```python
from build123d import *

# Parameters (mm, degrees)
F0_R     = 1.5875
F1_DEPTH = 1.778
F3_DEPTH = 9.525


with BuildPart() as f1:
    # F0 (on Top) → F1 (new body)
    with BuildSketch(Plane.XY):
        with BuildLine():
            Line((0, 53.34), (0, 0))
            Line((0, 0), (66.04, 0))
            Line((66.04, 0), (66.04, 2.54))
            Line((66.04, 2.54), (66.04, 6.0325))
            ThreePointArc((66.04, 6.0325), (64.4525, 7.62), (66.04, 9.2075))
            ThreePointArc((66.04, 9.2075), (67.1625320151, 8.7425320151), (67.6275, 7.62))
            Line((67.6275, 7.62), (68.58, 7.62))
            Line((68.58, 7.62), (68.58, 37.846))
            Line((68.58, 37.846), (66.04, 40.386))
            Line((66.04, 40.386), (66.04, 51.816))
            Line((66.04, 51.816), (64.516, 53.34))
            Line((64.516, 53.34), (0, 53.34))
        make_face()
        with Locations((13.97, 2.54)):
            Circle(F0_R, mode=Mode.SUBTRACT)
        with BuildLine():
            ThreePointArc((13.6525, 50.8), (15.24, 52.3875), (16.8275, 50.8))
            ThreePointArc((16.8275, 50.8), (15.24, 49.2125), (13.6525, 50.8))
        make_face(mode=Mode.SUBTRACT)
        with BuildLine():
            ThreePointArc((67.6275, 34.1701958202), (67.1625320151, 33.0476638051), (66.04, 32.5826958202))
            ThreePointArc((66.04, 32.5826958202), (64.9174679849, 35.2927278354), (67.6275, 34.1701958202))
        make_face(mode=Mode.SUBTRACT)
        with BuildLine():
            Line((66.04, 6.0325), (66.04, 2.54))
            Line((66.04, 2.54), (68.58, 5.08))
            Line((68.58, 5.08), (68.58, 7.62))
            Line((68.58, 7.62), (67.6275, 7.62))
            ThreePointArc((67.6275, 7.62), (67.1625320151, 6.4974679849), (66.04, 6.0325))
        make_face()
    extrude(amount=F1_DEPTH)

    # F2 (on face) → F3 (join)
    with BuildSketch(Plane.XY.offset(1.778)):
        Polygon((0, 32.385), (9.525, 32.385), (9.525, 45.085), (-6.35, 45.085), (-6.35, 32.385), align=None)
        Polygon((0, 3.175), (11.43, 3.175), (11.43, 12.065), (-1.905, 12.065), (-1.905, 3.175), align=None)
    extrude(amount=F3_DEPTH)


solid = f1.part
```
Geometry: final body of the model. Coordinates: model frame, mm. A direction names the side the tool comes from. Round coordinates to 2 decimals unless told otherwise and drop trailing zeros. Order: outer loops, then holes, each group sorted by start corner. A loop starts at its lowest first (then second) coordinate and runs counter-clockwise, first axis right, second up. Notation, with made-up numbers: (52, 31) - (62, 31) arc R7 cw to (62, 35) - close; hole circle Ø8 at (58.25, 46). An arc over 180 degrees is marked (long way). Write item = value, one per line. Start each with the question number.
Q1. Pull-direction query (Y, two-part tool) for faces 5 (the flat face through (1, 32.385, 6)), 6 (the flat face through (1, 39, 11.303)), 7 (the flat face through (5, 12.065, 6)), 8 (the flat face through (67.328, 39.098, 0.877)); classes: +Y half, -Y half, draft (parallel to the pull), parting line (faces both ways), or undercut.
Q2. Cut plane D-D on z = 1. Return the cut outline in (x, y) (1 decimal).
Q3. Ray query, line 1 (X direction, y = 50.8, z = 1.45); line 2 (Y direction, x = 13.97, z = 0.9); line 3 (X direction, y = 10, z = 4) (3 decimals). Return the intervals inside material, ascending. Write a range as from..to.
Q4. Access query for faces 1 (the flat face through (9.525, 39, 6)), 2 (the flat face through (5, 3.175, 6)), 3 (the flat face through (-3, 39, 1.778)), 4 (the flat face through (66.04, 1, 1)). Directions: +Z, -Z, +X, -X, +Y, -Y. A direction counts if a zero-diameter tool reaches every point of the face in a straight line with its end or side. Return the directions, or none.
Q5. Pin query (flat end, axial travel): pin 1 (2 mm diameter, centred on y = 47, z = 0.5, fed in from +X); pin 2 (0.9 mm diameter, centred on y = 24, z = 1, fed in from -X); pin 3 (3 mm diameter, centred on x = -3, y = 35.5, fed in from -Z). Return the tip coordinate at first contact, or that it passes through.
Q6. Cut plane B-B on z = 4.5. Return the cut outline in (x, y) (3 decimals), and give its area (3 significant figures).
Q7. Cut plane C-C on y = 43. Return the cut outline in (x, z) (3 decimals), and give its area (3 significant figures).
Q8. Cut plane A-A on y = 50.8. Return the cut outline in (x, z).
Outcome:
q1.face_5 = undercut
q1.face_6 = draft
q1.face_7 = undercut
q1.face_8 = +Y half
q2.outline = (0, 0) - (66, 0) - (66, 2.5) - (68.6, 5.1) - (68.6, 37.8) - (66, 40.4) - (66, 51.8) - (64.5, 53.3) - (0, 53.3) - close; hole circle Ø3.2 at (14, 2.5); hole circle Ø3.2 at (15.2, 50.8); hole circle Ø3.2 at (66, 7.6); hole circle Ø3.2 at (66, 34.2)
q3.line_1 = 0..13.65, 16.83..66.04
q3.line_2 = 0..0.95, 4.13..49.85, 51.75..53.34
q3.line_3 = -1.905..11.43
q4.face_1 = +Z, +X, +Y
q4.face_2 = +Z, +X, -X, -Y
q4.face_3 = -Z, -X, +Y, -Y
q4.face_4 = +Z, -Z, +X, -Y
q5.pin_1 = 66.04
q5.pin_2 = 0
q5.pin_3 = 1.78
q6.outline = (-6.35, 32.385) - (9.525, 32.385) - (9.525, 45.085) - (-6.35, 45.085) - close; (-1.905, 3.175) - (11.43, 3.175) - (11.43, 12.065) - (-1.905, 12.065) - close
q6.area = 320 mm^2
q7.outline = (-6.35, 1.778) - (0, 1.778) - (0, 0) - (66.04, 0) - (66.04, 1.778) - (9.525, 1.778) - (9.525, 11.303) - (-6.35, 11.303) - close
q7.area = 269 mm^2
q8.outline = (0, 0) - (13.65, 0) - (13.65, 1.78) - (0, 1.78) - close; (16.83, 0) - (66.04, 0) - (66.04, 1.78) - (16.83, 1.78) - close
